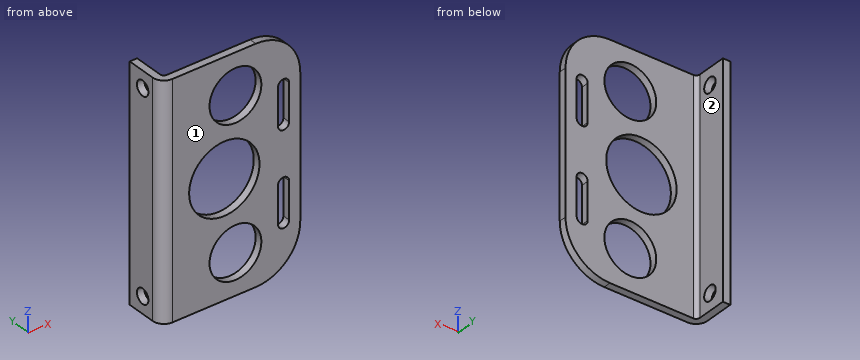
from build123d import *

# Parameters (mm, degrees)
EXTRUDE_1_DEPTH       = 31
SKETCH_2_R            = 2
CUT_EXTRUDE_1_DEPTH   = 49.396797415
SKETCH_3_R            = 9.5
SKETCH_3_R_2          = 7
CUT_EXTRUDE_2_DEPTH   = 50.479793856
FILLET_1_R            = 12
SHEET_START           = -31
SHEET_METAL_1_DEPTH   = 62
SHEET_METAL_1_2_DEPTH = 62


# Read off the part's stored shape, not the designer's step: 转换实体1
with BuildPart() as part:
    # Sketch 1 → 拉伸-薄壁1 (new, symmetric)
    with BuildSketch(Plane.XY):
        Polygon((0, 11), (0, 0), (37.5, 0), (37.5, 2), (2, 2), (2, 11), align=None)
    extrude(amount=EXTRUDE_1_DEPTH, both=True)

    # Sketch 2 → 切除-拉伸1 (cut, through all)
    with BuildSketch(Plane(origin=(2, 0, 0), x_dir=(0, 0, -1), z_dir=(1, 0, 0))):
        with Locations(Location((-26.5, 6.5, 0), (0, 0, 90))):
            Circle(SKETCH_2_R)
        with Locations(Location((26.5, 6.5, 0), (0, 0, 270))):
            Circle(SKETCH_2_R)
    extrude(amount=-CUT_EXTRUDE_1_DEPTH, mode=Mode.SUBTRACT)

    # 草图3 → 切除-拉伸2 (cut, through all)
    with BuildSketch(Plane(origin=(0, 2, 0), x_dir=(1, 0, 0), z_dir=(0, 1, 0))):
        with Locations(Location((17, 0, 0), (0, 0, 270))):
            Circle(SKETCH_3_R)
        with Locations(Location((20, 20, 0), (0, 0, 270))):
            Circle(SKETCH_3_R_2)
        with Locations(Location((20, -20, 0), (0, 0, 90))):
            Circle(SKETCH_3_R_2)
        with BuildLine():
            Line((34.5, -7.5), (34.5, -17.5))
            ThreePointArc((34.5, -17.5), (33, -19), (31.5, -17.5))
            Line((31.5, -17.5), (31.5, -7.5))
            ThreePointArc((31.5, -7.5), (33, -6), (34.5, -7.5))
        make_face()
        with BuildLine():
            Line((34.5, 7.5), (34.5, 17.5))
            ThreePointArc((34.5, 17.5), (33, 19), (31.5, 17.5))
            Line((31.5, 17.5), (31.5, 7.5))
            ThreePointArc((31.5, 7.5), (33, 6), (34.5, 7.5))
        make_face()
    extrude(amount=-CUT_EXTRUDE_2_DEPTH, mode=Mode.SUBTRACT)

    # 圆角1
    fillet_1_edges = [part.edges().sort_by_distance(p)[0] for p in [
        (37.5, 1, -31),
        (37.5, 1, 31),
    ]]
    fillet(fillet_1_edges, radius=FILLET_1_R)

    # Sheet Metal 1 outline → Sheet Metal 1 (cut)
    with BuildSketch(Plane.XY.offset(SHEET_START)):
        with BuildLine():
            ThreePointArc((3, 0), (0.878679656, 0.878679656), (0, 3))
            Line((0, 3), (0, 0))
            Line((0, 0), (3, 0))
        make_face()
    extrude(amount=SHEET_METAL_1_DEPTH, mode=Mode.SUBTRACT)

    # Sheet Metal 1 2 outline → Sheet Metal 1 2 (add)
    with BuildSketch(Plane.XY.offset(SHEET_START)):
        with BuildLine():
            ThreePointArc((3, 2), (2.292893219, 2.292893219), (2, 3))
            Line((2, 3), (2, 2))
            Line((2, 2), (3, 2))
        make_face()
    extrude(amount=SHEET_METAL_1_2_DEPTH)


solid = part.part
Could you check a few things on this model? Use its own coordinates, in mm. Face numbers are marked on the shaded views. A direction names the side the tool comes from. Round coordinates to 2 decimals unless told otherwise and drop trailing zeros. Loops run counter-clockwise (first coordinate to the right, second up) from the corner with the lowest first, then second, coordinate; pieces in that order, holes last. Notation, with made-up numbers: (-22, 5.25) -> (36, 5.25) arc R18 ccw to (36, 25.25) -> close; hole circle Ø4 at (3.25, 81). An arc over 180 degrees is marked (long way). Use CSV: the item, a comma, the result in double quotes.
(1) If I drill on probe 1 along Z at (x, y) = (1, 6.5); probe 2 along X at (y, z) = (0.5, 15.5); probe 3 along Z at (x, y) = (20.5, 1.5), over which ranges is the centre line in solid material (lowest first)? Write a range as [from, to].
Return value:
probe 1,"z = [-31, -28.5], [-24.5, 24.5], [28.5, 31]"
probe 2,"x = [1.34, 14.64], [25.36, 31.5], [34.5, 37.5]"
probe 3,"z = [-31, -26.98], [-13.02, -8.83], [8.83, 13.02], [26.98, 31]"
(2) Suppose I cut it at D-D on x = 17. Write out the boundary of the cut face in (y, z), plus the area to 3 significant figures.
Return value:
outline,"(0, -31) -> (2, -31) -> (2, -26.32) -> (0, -26.32) -> close; (0, -13.68) -> (2, -13.68) -> (2, -9.5) -> (0, -9.5) -> close; (0, 9.5) -> (2, 9.5) -> (2, 13.68) -> (0, 13.68) -> close; (0, 26.32) -> (2, 26.32) -> (2, 31) -> (0, 31) -> close"
area,"35.4 mm²"
(3) Suppose I cut it at A-A on y = 6.5. Write out the boundary of the cut face in (x, z), plus the area to 3 significant figures.
Return value:
outline,"(0, -31) -> (2, -31) -> (2, -28.5) -> (0, -28.5) -> close; (0, -24.5) -> (2, -24.5) -> (2, 24.5) -> (0, 24.5) -> close; (0, 28.5) -> (2, 28.5) -> (2, 31) -> (0, 31) -> close"
area,"108 mm²"
(4) Will these pins go through, and if not, where does the flat tip stop? pin 1 Ø6.5 at (y, z) = (8, 4.5) entering from +X; pin 2 Ø6 at (x, y) = (30.5, 4.5) entering from +Z; pin 3 Ø3 at (x, z) = (18, -14.5) entering from +Y.
Return value:
pin 1,"stops at x = 2"
pin 2,"stops at z = 30.53"
pin 3,"stops at y = 2"
(5) For the marked faces 1 and 2, which set-ups out of +Z, -Z, +X, -X, +Y, -Y let a thin tool reach every point of the face, with its end or its side?
Return value:
face 1,"+Z, -Z, +X, -X, -Y"
face 2,"+Z, -Z, +X, +Y"
(6) Suppose I cut it at C-C on z = 11. Write out the boundary of the cut face in (x, y).
Return value:
outline,"(0, 3) arc R3 ccw to (3, 0) -> (31.5, 0) -> (31.5, 2) -> (3, 2) arc R1 cw to (2, 3) -> (2, 11) -> (0, 11) -> close; (34.5, 0) -> (37.5, 0) -> (37.5, 2) -> (34.5, 2) -> close"
(7) Suppose I cut it at B-B on x = 33. Write out the boundary of the cut face in (y, z), plus the area to 3 significant figures.
Return value:
outline,"(0, -28.37) -> (2, -28.37) -> (2, -19) -> (0, -19) -> close; (0, -6) -> (2, -6) -> (2, 6) -> (0, 6) -> close; (0, 19) -> (2, 19) -> (2, 28.37) -> (0, 28.37) -> close"
area,"61.5 mm²"
